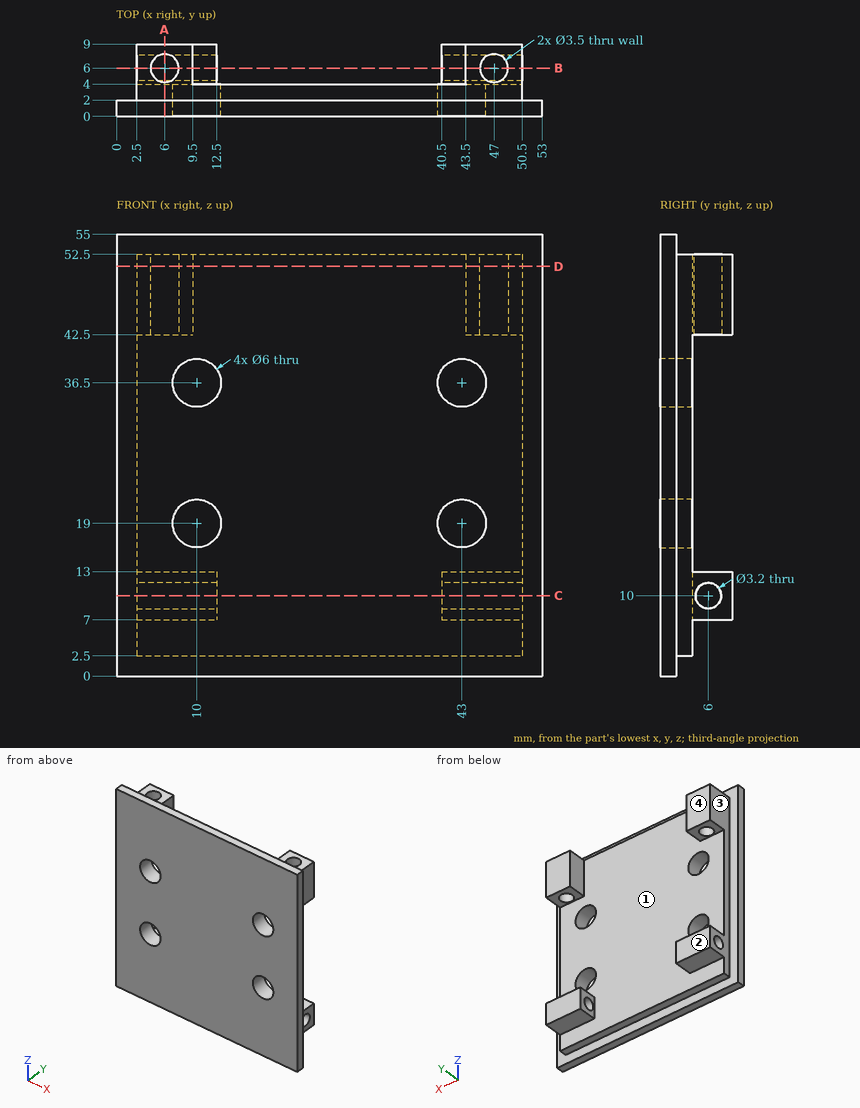
Input: dimensioned drawing with shaded views. Units: mm. Origin: part minimum x, y, z. A direction names the side the tool comes from. Give positions to 0.01 mm unless a question says otherwise; leave off trailing zeros. Order: outer loops, then holes, each group sorted by start corner. A loop starts at its lowest first (then second) coordinate and runs counter-clockwise, first axis right, second up. Notation, with made-up numbers: (9.25, 70.5) -> (20.25, 70.5) arc R24 ccw to (20.25, 106.5) -> close; hole circle Ø2 at (35, -32). An arc over 180 degrees is marked (long way). Answer as a JSON object with one key per item and string values.
Q1. Section C-C (z = 10). Output: boundary loops of the cut face in (x, y), plus the area to 3 significant figures.
Entries:
{"outline": "(0, 0) -> (53, 0) -> (53, 2) -> (50.5, 2) -> (50.5, 4.4) -> (40.5, 4.4) -> (40.5, 4) -> (12.5, 4) -> (12.5, 4.4) -> (2.5, 4.4) -> (2.5, 2) -> (0, 2) -> close; (2.5, 7.6) -> (12.5, 7.6) -> (12.5, 9) -> (2.5, 9) -> close; (40.5, 7.6) -> (50.5, 7.6) -> (50.5, 9) -> (40.5, 9) -> close", "area": "238 mm^2"}
Q2. Access query for the marked faces 3 and 4. Directions: +Z, -Z, +X, -X, +Y, -Y. A direction counts if a zero-diameter tool reaches every point of the face in a straight line with its end or side. Return the directions, or none.
Entries:
{"face 3": "+Z, -Z, -X, +Y", "face 4": "+Z, -Z, +X, -X, +Y"}
Q3. Section B-B (y = 6). State how many separate pieces and enclosed holes the cut face has, plus the area to 3 significant figures.
Entries:
{"separate pieces": "8", "enclosed holes": "0", "area": "126 mm^2"}
Q4. Section A-A (x = 6). Output: boundary loops of the cut face in (y, z).
Entries:
{"outline": "(0, 0) -> (2, 0) -> (2, 2.5) -> (4, 2.5) -> (4, 7) -> (9, 7) -> (9, 13) -> (4, 13) -> (4, 42.5) -> (4.25, 42.5) -> (4.25, 52.5) -> (2, 52.5) -> (2, 55) -> (0, 55) -> close; (7.75, 42.5) -> (9, 42.5) -> (9, 52.5) -> (7.75, 52.5) -> close; hole circle Ø3.2 at (6, 10)"}
Q5. Draft query along Z for the marked faces 1 and 2. Return one class per face: released by +Z, released by -Z, zero draft, split by the parting line, or undercut.
Entries:
{"face 1": "undercut", "face 2": "zero draft"}
Q6. Section D-D (z = 51). Output: boundary loops of the cut face in (x, y), plus the area to 3 significant figures.
Entries:
{"outline": "(0, 0) -> (53, 0) -> (53, 2) -> (50.5, 2) -> (50.5, 9) -> (43.5, 9) -> (43.5, 4) -> (9.5, 4) -> (9.5, 9) -> (2.5, 9) -> (2.5, 2) -> (0, 2) -> close; hole circle Ø3.5 at (6, 6); hole circle Ø3.5 at (47, 6)", "area": "253 mm^2"}
Q7. Material intervals for probe 1 along X at (y, z) = (1.55, 19); probe 2 along X at (y, z) = (4.25, 10.5); probe 3 along Y at (x, z) = (6, 50), sorted ascending.
Entries:
{"probe 1": "x = 0 to 7, 13 to 40, 46 to 53", "probe 2": "x = 2.5 to 12.5, 40.5 to 50.5", "probe 3": "y = 0 to 4.25, 7.75 to 9"}
Q8. First-contact query: pin 1 (7 mm diameter, centred on x = 43, z = 19, fed in from +Y); pin 2 (2.5 mm diameter, centred on x = 45, y = 6.5, fed in from -Z); pin 3 (3 mm diameter, centred on y = 5.5, z = 46.5, fed in from +X). Flat tips, straight axial feed; report the tip coordinate or a pass-through.
Entries:
{"pin 1": "stops at y = 4", "pin 2": "stops at z = 7", "pin 3": "stops at x = 50.5"}
